The drawing under review shows one solid part. Ordinate dimensions are in mm from its lowest x, y, z. Give positions to 0.01 mm unless a question says otherwise; leave off trailing zeros. Loops run counter-clockwise (first coordinate to the right, second up) from the corner with the lowest first, then second, coordinate; pieces in that order, holes last.
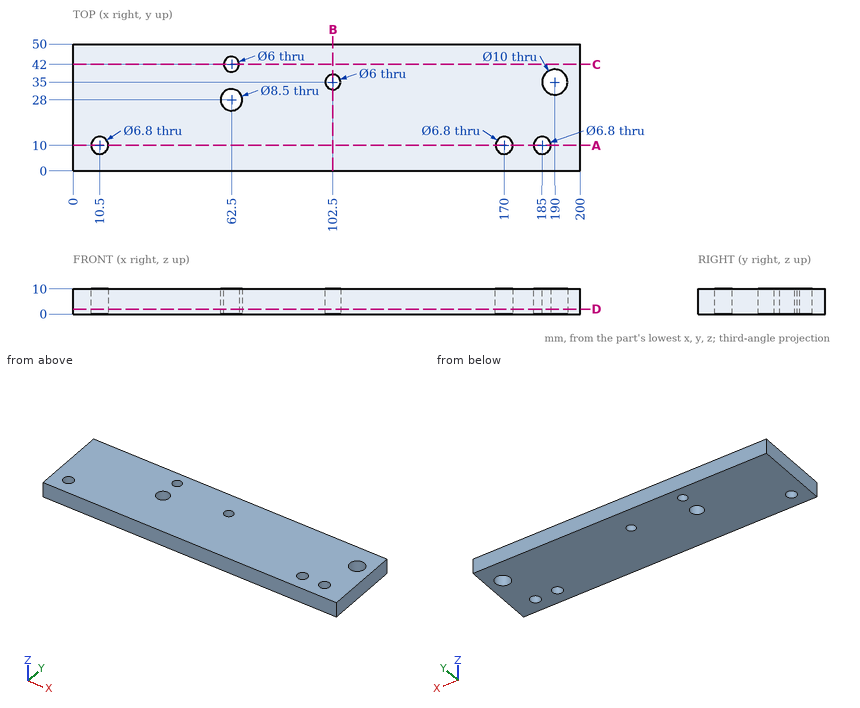
Item 1: Take a section at D-D on z = 2. Give the boundary of the cut face in (x, y), and give its area (3 significant figures).
Answer:
outline: (0, 0) - (200, 0) - (200, 50) - (0, 50) - close; hole circle Ø6.8 at (10.5, 10); hole circle Ø8.5 at (62.5, 28); hole circle Ø6 at (62.5, 42); hole circle Ø6 at (102.5, 35); hole circle Ø6.8 at (170, 10); hole circle Ø6.8 at (185, 10); hole circle Ø10 at (190, 35)
area: 9,700 mm2
Item 2: Clearance check with a flat-ended pin moving along its axis: pin 1 Ø5 at (x, y) = (102.5, 35) entering from +Z. State where the tip first meets the part, or that it passes through.
Answer:
pin 1: passes through
Item 3: Take a section at A-A on y = 10. Give the boundary of the cut face in (x, z).
Answer:
outline: (0, 0) - (7.1, 0) - (7.1, 10) - (0, 10) - close; (13.9, 0) - (166.6, 0) - (166.6, 10) - (13.9, 10) - close; (173.4, 0) - (181.6, 0) - (181.6, 10) - (173.4, 10) - close; (188.4, 0) - (200, 0) - (200, 10) - (188.4, 10) - close
Item 4: Take a section at C-C on y = 42. Give the boundary of the cut face in (x, z).
Answer:
outline: (0, 0) - (59.5, 0) - (59.5, 10) - (0, 10) - close; (65.5, 0) - (200, 0) - (200, 10) - (65.5, 10) - close
Item 5: For L1, parallel to Y at x = 62.5, z = 2.5; L2, parallel to X at y = 10.5, z = 6; L3, parallel to Y at x = 64.5, z = 9.25, list the stretches that pass through material, from the lowest coordinate up.
Answer:
L1: y = 0 to 23.75, 32.25 to 39, 45 to 50
L2: x = 0 to 7.14, 13.86 to 166.64, 173.36 to 181.64, 188.36 to 200
L3: y = 0 to 24.25, 31.75 to 39.76, 44.24 to 50
Item 6: Take a section at B-B on x = 102.5. Give the boundary of the cut face in (y, z), and give its area (3 significant figures).
Answer:
outline: (0, 0) - (32, 0) - (32, 10) - (0, 10) - close; (38, 0) - (50, 0) - (50, 10) - (38, 10) - close
area: 440 mm2
